Part print with two shaded views. Sizes in mm from the minimum x, y, z corner. Give positions to 0.01 mm unless a question says otherwise; leave off trailing zeros. Loops run counter-clockwise (first coordinate to the right, second up) from the corner with the lowest first, then second, coordinate; pieces in that order, holes last. Notation, with made-up numbers: M 34,22.25 L 92,22.25 A27 cw 92,60.25 Z; hole C 26,49.25 d7. An arc over 180 degrees is marked long. Answer as a JSON object with one key per item and string values. Group by question number.
1. Drop a flat-ended pin along its axis: pin 1 Ø1.3 at (x, y) = (5.08, 19.22) entering from -Z. Give the stop position or say it passes through.
2. Slice it at A-A (y = 12.15). List the corners of the cut face in (x, z).
3. Slice it at D-D (x = 19.5). List the corners of the cut face in (y, z) (3 decimals).
4. Mould opens along Y. For the marked faces 1, 2 and 3 say: released by +Y, released by -Y, zero draft, split by the parting line, or undercut.
5. Slice it at C-C (z = 0.5). List the corners of the cut face in (x, y), then the cut area to 3 significant figures.
6. Drill centre lines: line 1 along Y through (x, z) = (19.25, 0.2); line 2 along X through (y, z) = (18.5, 0.9); line 3 along Y through (x, z) = (12.15, 1.55). Where is each one in solid material? Low to high. Write a range as [from, to].
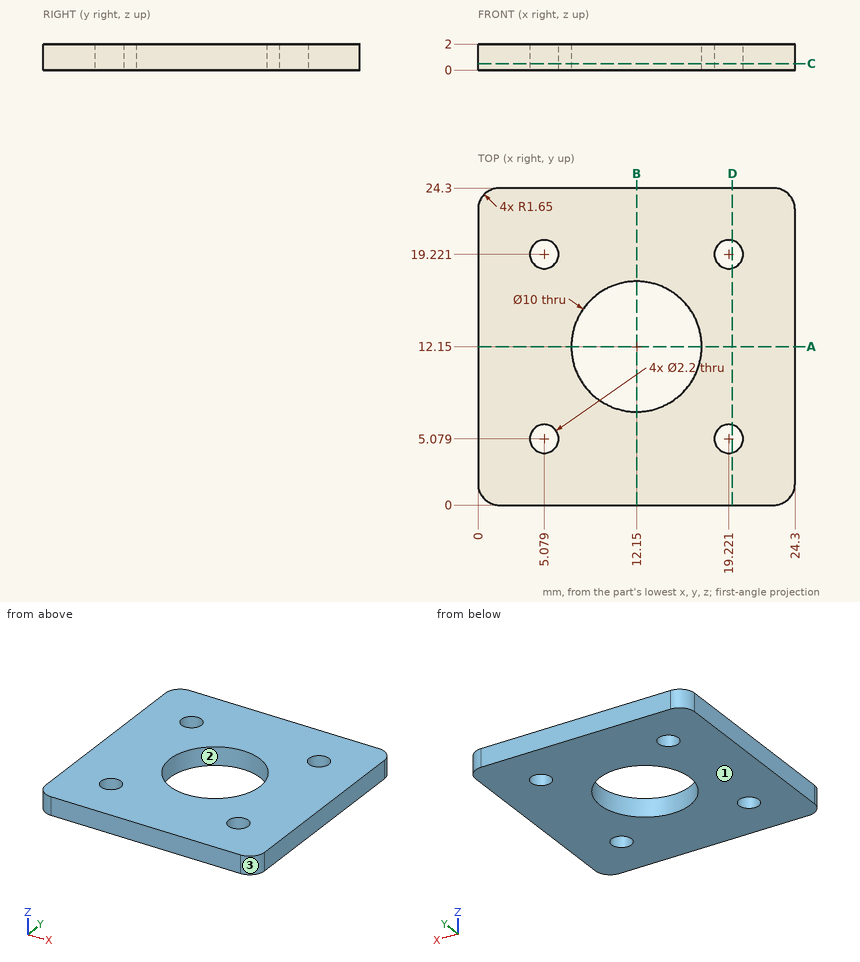
Established:
{
 "1": {"pin 1": "passes through"},
 "2": {"outline": "M 0,0 L 7.15,0 L 7.15,2 L 0,2 Z; M 17.15,0 L 24.3,0 L 24.3,2 L 17.15,2 Z"},
 "3": {"outline": "M 0,0 L 4.015,0 L 4.015,2 L 0,2 Z; M 6.143,0 L 18.157,0 L 18.157,2 L 6.143,2 Z; M 20.285,0 L 24.3,0 L 24.3,2 L 20.285,2 Z"},
 "4": {"face 1": "zero draft", "face 2": "undercut", "face 3": "released by -Y"},
 "5": {"outline": "M 0,1.65 A1.65 ccw 1.65,0 L 22.65,0 A1.65 ccw 24.3,1.65 L 24.3,22.65 A1.65 ccw 22.65,24.3 L 1.65,24.3 A1.65 ccw 0,22.65 Z; hole C 5.08,5.08 d2.2; hole C 5.08,19.22 d2.2; hole C 12.15,12.15 d10; hole C 19.22,5.08 d2.2; hole C 19.22,19.22 d2.2", "area": "494 mm^2"},
 "6": {"line 1": "y = [0, 3.98], [6.18, 18.12], [20.32, 24.3]", "line 2": "x = [0, 4.25], [5.91, 18.39], [20.05, 24.3]", "line 3": "y = [0, 7.15], [17.15, 24.3]"}
}
